Read the model definition and answer for the solid it produces. Units are mm, in the model's axes. A direction names the side the tool comes from. Coordinates: 2 decimals unless noted, no trailing zeros. Write each loop counter-clockwise with the first axis right and the second up, starting at its lowest first coordinate (ties: lowest second). Pieces come first, ordered by that corner, then holes. Notation, with made-up numbers: M 58,-28.75 L 89,-28.75 A17 ccw 89,-0.75 Z; hole C 77.25,80.5 d11. An arc over 180 degrees is marked long. Write item = value, one per line.
from build123d import *

# Parameters (mm, degrees)
SCHIZZO1_R                   = 2.15
ESTRUSIONE_ESTRUSIONE1_DEPTH = 100


with BuildPart() as part:
    # Schizzo1 → Estrusione-Estrusione1 (new body)
    with BuildSketch(Plane(origin=(0, 0, 0), x_dir=(-1, 0, 0), z_dir=(0, 0, -1))):
        with BuildLine():
            Line((8.2, 2.5), (9, 2.5))
            ThreePointArc((9, 2.5), (9.707106781, 2.792893219), (10, 3.5))
            Line((10, 3.5), (10, 9))
            ThreePointArc((10, 9), (9.707106781, 9.707106781), (9, 10))
            Line((9, 10), (3.5, 10))
            ThreePointArc((3.5, 10), (2.792893219, 9.707106781), (2.5, 9))
            Line((2.5, 9), (2.5, 8.2))
            Line((2.5, 8.2), (4.512994231, 8.2))
            ThreePointArc((4.512994231, 8.2), (5.436873764, 7.582683432), (5.220101013, 6.492893219))
            Line((5.220101013, 6.492893219), (2.670101013, 3.942893219))
            ThreePointArc((2.670101013, 3.942893219), (2.345677664, 3.726120467), (1.962994231, 3.65))
            Line((1.962994231, 3.65), (-1.962994231, 3.65))
            ThreePointArc((-1.962994231, 3.65), (-2.345677664, 3.726120467), (-2.670101013, 3.942893219))
            Line((-2.670101013, 3.942893219), (-5.220101013, 6.492893219))
            ThreePointArc((-5.220101013, 6.492893219), (-5.436873764, 7.582683432), (-4.512994231, 8.2))
            Line((-4.512994231, 8.2), (-2.5, 8.2))
            Line((-2.5, 8.2), (-2.5, 9))
            ThreePointArc((-2.5, 9), (-2.792893219, 9.707106781), (-3.5, 10))
            Line((-3.5, 10), (-9, 10))
            ThreePointArc((-9, 10), (-9.707106781, 9.707106781), (-10, 9))
            Line((-10, 9), (-10, 3.5))
            ThreePointArc((-10, 3.5), (-9.707106781, 2.792893219), (-9, 2.5))
            Line((-9, 2.5), (-8.2, 2.5))
            Line((-8.2, 2.5), (-8.2, 4.512994231))
            ThreePointArc((-8.2, 4.512994231), (-7.582683432, 5.436873764), (-6.492893219, 5.220101013))
            Line((-6.492893219, 5.220101013), (-3.942893219, 2.670101013))
            ThreePointArc((-3.942893219, 2.670101013), (-3.726120467, 2.345677664), (-3.65, 1.962994231))
            Line((-3.65, 1.962994231), (-3.65, -1.962994231))
            ThreePointArc((-3.65, -1.962994231), (-3.726120467, -2.345677664), (-3.942893219, -2.670101013))
            Line((-3.942893219, -2.670101013), (-6.492893219, -5.220101013))
            ThreePointArc((-6.492893219, -5.220101013), (-7.582683432, -5.436873764), (-8.2, -4.512994231))
            Line((-8.2, -4.512994231), (-8.2, -2.5))
            Line((-8.2, -2.5), (-9, -2.5))
            ThreePointArc((-9, -2.5), (-9.707106781, -2.792893219), (-10, -3.5))
            Line((-10, -3.5), (-10, -9))
            ThreePointArc((-10, -9), (-9.707106781, -9.707106781), (-9, -10))
            Line((-9, -10), (-3.5, -10))
            ThreePointArc((-3.5, -10), (-2.792893219, -9.707106781), (-2.5, -9))
            Line((-2.5, -9), (-2.5, -8.2))
            Line((-2.5, -8.2), (-4.512994231, -8.2))
            ThreePointArc((-4.512994231, -8.2), (-5.436873764, -7.582683432), (-5.220101013, -6.492893219))
            Line((-5.220101013, -6.492893219), (-2.670101013, -3.942893219))
            ThreePointArc((-2.670101013, -3.942893219), (-2.345677664, -3.726120467), (-1.962994231, -3.65))
            Line((-1.962994231, -3.65), (1.962994231, -3.65))
            ThreePointArc((1.962994231, -3.65), (2.345677664, -3.726120467), (2.670101013, -3.942893219))
            Line((2.670101013, -3.942893219), (5.220101013, -6.492893219))
            ThreePointArc((5.220101013, -6.492893219), (5.436873764, -7.582683432), (4.512994231, -8.2))
            Line((4.512994231, -8.2), (2.5, -8.2))
            Line((2.5, -8.2), (2.5, -9))
            ThreePointArc((2.5, -9), (2.792893219, -9.707106781), (3.5, -10))
            Line((3.5, -10), (9, -10))
            ThreePointArc((9, -10), (9.707106781, -9.707106781), (10, -9))
            Line((10, -9), (10, -3.5))
            ThreePointArc((10, -3.5), (9.707106781, -2.792893219), (9, -2.5))
            Line((9, -2.5), (8.2, -2.5))
            Line((8.2, -2.5), (8.2, -4.512994231))
            ThreePointArc((8.2, -4.512994231), (7.582683432, -5.436873764), (6.492893219, -5.220101013))
            Line((6.492893219, -5.220101013), (3.942893219, -2.670101013))
            ThreePointArc((3.942893219, -2.670101013), (3.726120467, -2.345677664), (3.65, -1.962994231))
            Line((3.65, -1.962994231), (3.65, 1.962994231))
            ThreePointArc((3.65, 1.962994231), (3.726120467, 2.345677664), (3.942893219, 2.670101013))
            Line((3.942893219, 2.670101013), (6.492893219, 5.220101013))
            ThreePointArc((6.492893219, 5.220101013), (7.582683432, 5.436873764), (8.2, 4.512994231))
            Line((8.2, 4.512994231), (8.2, 2.5))
        make_face()
        Circle(SCHIZZO1_R, mode=Mode.SUBTRACT)
    extrude(amount=-ESTRUSIONE_ESTRUSIONE1_DEPTH)


solid = part.part
Item 1: Flat-ended cylindrical pins translate along their axes: pin 1 (10 mm diameter, centred on x = 3, y = -3, fed in from -Z); pin 2 (1.2 mm diameter, centred on y = -1, z = 44.5, fed in from +X); pin 3 (3 mm diameter, centred on x = 0.5, z = 27, fed in from -Y); pin 4 (0.6 mm diameter, centred on x = -3, z = 52, fed in from -Y). Find the tip coordinate at first contact, or state that the pin passes through.
Worked answers:
pin_1 = 0
pin_2 = 3.65
pin_3 = -3.65
pin_4 = -9.98
Item 2: Find section A-A (x = 0). Determine the outline of the cut face in (y, z).
Worked answers:
outline = M -3.65,0 L -2.15,0 L -2.15,100 L -3.65,100 Z; M 2.15,0 L 3.65,0 L 3.65,100 L 2.15,100 Z
Item 3: Which of the six approach directions +Z, -Z, +X, -X, +Y, -Y give full straight-line access (tool end or side, diameter ignored) to faces 1 (the face through (0.1, 2.4, 100)), 2 (the face through (10, 6, 49)), 3 (the face through (-3.65, 0, 49)), 4 (the face through (4, 8.2, 49)), 5 (the face through (0, 3.65, 49))?
Worked answers:
face_1 = +Z, +X, -X, +Y, -Y
face_2 = +Z, -Z, +X, +Y, -Y
face_3 = +Z, -Z, -X
face_4 = +Z, -Z
face_5 = +Z, -Z, +Y
Item 4: For a pull along Y with two mould halves and no side action, classify faces 6 (the face through (-10, -6, 49)), 7 (the face through (6, 10, 49)), 8 (the face through (-3, 8.2, 49)), 9 (the face through (3.963, -5.236, 49.3)) as released by +Y, released by -Y, zero draft, split by the parting line, or undercut.
Worked answers:
face_6 = zero draft
face_7 = released by +Y
face_8 = undercut
face_9 = undercut
Item 5: Consider line 1 along Y through (x, z) = (-6.5, 28.5); line 2 along Y through (x, z) = (7, 26); line 3 along X through (y, z) = (-4, 74). Determine where each line is inside the solid, lowest interval first. Write a range as from..to.
Worked answers:
line_1 = -10..-5.23, 5.23..10
line_2 = -10..-5.49, 5.49..10
line_3 = -10..-8.2, -5.27..-2.73, 2.73..5.27, 8.2..10
